Here's the drawing with two shaded views (mm, measured from the low corner). I have some questions. A direction names the side the tool comes from. Give positions to 0.01 mm unless a question says otherwise; leave off trailing zeros. Loops run counter-clockwise (first coordinate to the right, second up) from the corner with the lowest first, then second, coordinate; pieces in that order, holes last. Notation, with made-up numbers: (54.5, -37) -> (95.5, -37) arc R32 cw to (95.5, -1) -> close; hole circle Ø3 at (-31, 8). An arc over 180 degrees is marked (long way). Write each question's results on one line, items separated by ' | '. Start each with the question number.
Q1. If I drill on line 1 along Y through (x, z) = (2.25, 6.25); line 2 along Z through (x, y) = (4.25, 7.5); line 3 along Y through (x, z) = (5.25, 6.25), over which ranges is the centre line in solid material (lowest first)?
Q2. We'd pull the mould along X, two halves only. Please class the marked faces 4, 5, 6 and 7: released by +X, released by -X, zero draft, split by the parting line, or undercut.
Q3. If we section it at A-A, the plane y = 7.25: List the corners of the cut face in (x, z) for me, plus the area to 3 significant figures.
Q4. Will these pins go through, and if not, where does the flat tip stop? P1, Ø2, axis at x = 2.5, y = 7, coming from the +Z side; P2, Ø1, axis at y = 13.5, z = 1.5, coming from the +X side (1 decimal).
Q5. Which directions (+Z, -Z, +X, -X, +Y, -Y) give clear straight access to the entire face, cutting with the end or side of a thin tool? Please do the marked faces 1, 2 and 3.
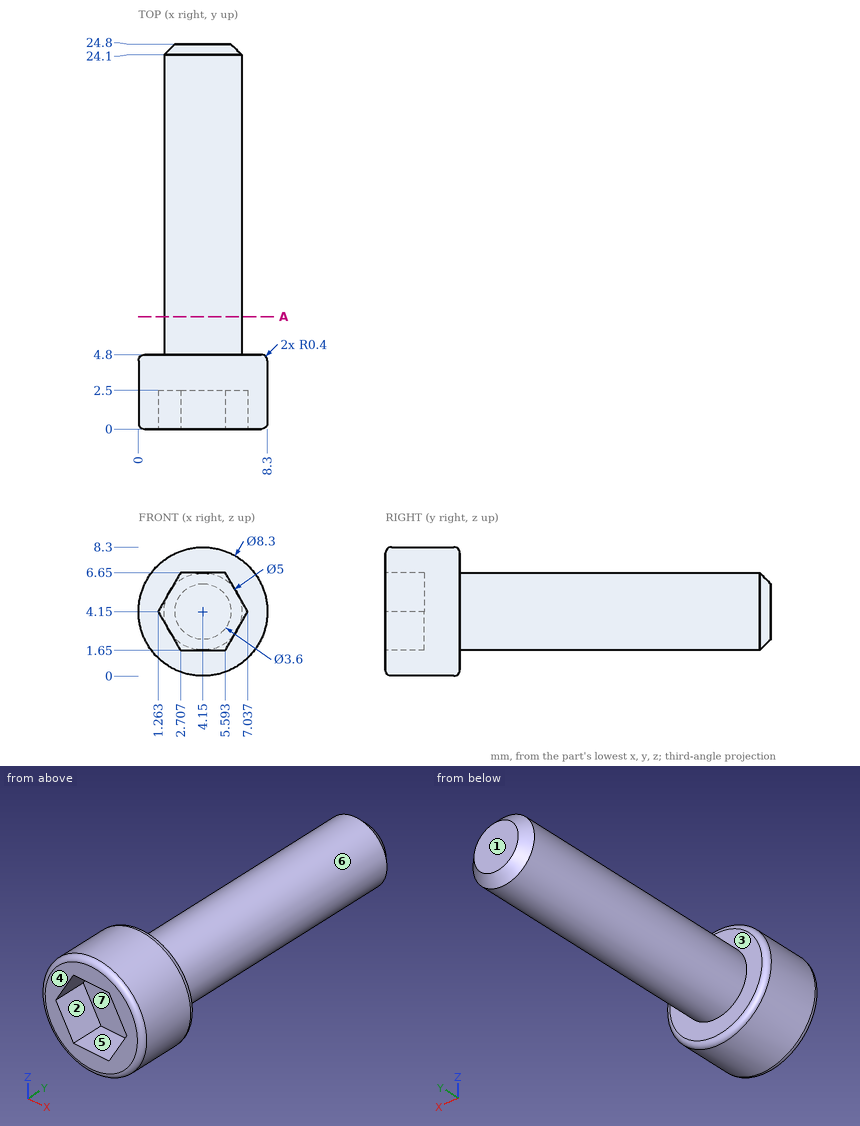
Final values:
1) line 1: y = 0 to 4.8 | line 2: z = 1.65 to 6.65 | line 3: y = 2.5 to 24.23
2) face 4: zero draft | face 5: undercut | face 6: split by the parting line | face 7: undercut
3) outline: circle Ø5 at (4.15, 4.15) | area: 19.6 mm²
4) P1: stops at z = 6.56 | P2: stops at x = 5.4
5) face 1: +Z, -Z, +X, -X, +Y | face 2: -Y | face 3: +Y
